Can you work these out from the model? Positions are in its coordinate system, mm. Face numbers are marked on the shaded views. A direction names the side the tool comes from. Round coordinates to 2 decimals unless told otherwise and drop trailing zeros. Loops run counter-clockwise (first coordinate to the right, second up) from the corner with the lowest first, then second, coordinate; pieces in that order, holes last. Notation, with made-up numbers: M -37,86 L 11,86 A26 cw 11,100 Z; hole C 24,72 d10. An arc over 180 degrees is marked long. Return JSON: item names as keys, results as strings.
Autodesk Inventor part; units mm, degrees
ref_plane "YZ Plane" through (0, 0, 0) normal (1, 0, 0) x (0, 1, 0)
ref_plane "XZ Plane" through (0, 0, 0) normal (0, 1, 0) x (-1, 0, 0)
ref_plane "XY Plane" through (0, 0, 0) normal (0, 0, 1) x (1, 0, 0)
sketch "Sketch1" plane through (0, 0, 0) normal (0, 1, 0) x (-1, 0, 0)
  line L0 (0, 0) -> (48.3, 0)
  line L1 (48.3, 0) -> (48.3, -15)
  line L2 (48.3, -15) -> (0, -15)
  line L3 (0, -15) -> (0, 0)
  circle A0 centre (48.3, 0) radius 1.5
  circle A1 centre (48.3, -15) radius 1.5
  line L4 (48.3, -15) -> (52.3, -15)
  line L5 (52.3, -15) -> (52.3, -17.5)
  line L6 (52.3, -17.5) -> (48.3, -17.5)
  line L7 (48.3, -17.5) -> (48.3, -15)
  line L8 (0, 0) -> (-4, 0)
  line L9 (-4, 0) -> (-4, 2.5)
  line L10 (-4, 2.5) -> (0, 2.5)
  line L11 (0, 2.5) -> (0, 0)
  line L12 (-4, 2.5) -> (52.3, 2.5)
  line L13 (52.3, 2.5) -> (52.3, -17.5)
  line L14 (52.3, -17.5) -> (-4, -17.5)
  line L15 (-4, -17.5) -> (-4, 2.5)
  line L16 (0, -2.5) -> (0, -12.5)
  circle A2 centre (0, -12.5) radius 2
  circle A3 centre (0, -2.5) radius 2
  point P0 (0, -7.5)
  dimension "d0" = 48.3
  dimension "d1" = 15
  dimension "d2" = 3
  dimension "d3" = 3
  dimension "d6" = 4
  dimension "d7" = 2.5
  dimension "d8" = 4
  dimension "d9" = 2.5
  dimension "d33" = 10
  dimension "d34" = 4
  dimension "d35" = 4
extrude "Extrusion1" add sketch "Sketch1" along normal blind 4 contours L11 L12 L13 L4 A1 L1 A0 L0 | L0 A0 L1 A1 L2 L3 A2 A3 | L3 A3 A2 L2 A1 L7 L14 L15 L8 | L8 L9 L10 L11 | L7 A1 L4 L5 L6
sketch "Sketch2" plane through (0, 4, 0) normal (0, 1, 0) x (1, 0, 0)
  line L0 (4, -2.5) -> (4, 17.5)
  line L1 (4, -2.5) -> (-14.15, -2.5)
  line L2 (-14.15, -2.5) -> (-14.15, 7.5)
  line L3 (-14.15, 7.5) -> (4, 7.5)
  line L4 (4, 7.5) -> (4, -2.5)
  circle A0 centre (-14.15, 7.5) radius 5
  circle A1 centre (-14.15, 7.5) radius 3.15
  point P0 (0, 0)
  dimension "d12" = 18.15
  dimension "d13" = 10
  dimension "d14" = 10
  dimension "d19" = 6.3
extrude "Extrusion2" add sketch "Sketch2" along normal blind 4 and the other way blind 2.5 contours A0 L2 A1 L3 | L3 A1 L2 A0
extrude "Extrusion3" cut sketch "Sketch2" against normal blind 4 contours A1 L2 L3 | L3 L2 A1
fillet "Fillet2" radius 4 1 edges at (-19.15, 4, -7.5)
sketch "Sketch3" plane through (0, 4, 0) normal (0, 1, 0) x (1, 0, 0)
  line L0 (4, 17.5) -> (-52.3, 17.5)
  line L1 (-52.3, 17.5) -> (-40.3, 17.5)
  line L2 (-40.3, 17.5) -> (-40.3, 12.5)
  line L3 (-40.3, 12.5) -> (-52.3, 12.5)
  line L4 (-52.3, 12.5) -> (-52.3, 17.5)
  line L5 (-52.3, -2.5) -> (4, -2.5)
  line L6 (-52.3, -2.5) -> (-40.3, -2.5)
  line L7 (-40.3, -2.5) -> (-40.3, 2.5)
  line L8 (-40.3, 2.5) -> (-52.3, 2.5)
  line L9 (-52.3, 2.5) -> (-52.3, -2.5)
  line L10 (-40.3, 2.5) -> (-25.3, 2.5)
  line L11 (-25.3, 2.5) -> (-25.3, 12.5)
  line L12 (-25.3, 12.5) -> (-40.3, 12.5)
  line L13 (-40.3, 12.5) -> (-40.3, 2.5)
  point P0 (0, 0)
  dimension "d25" = 12
  dimension "d26" = 5
  dimension "d27" = 12
  dimension "d28" = 5
  dimension "d29" = 15
extrude "Extrusion4" cut sketch "Sketch3" against normal blind 4 contours L12 L11 L10 L13
fillet "Fillet3" radius 2 4 edges at (-52.3, 2, 2.5) (4, 2, 2.5) (4, 2, -17.5) (-52.3, 2, -17.5)
sketch "Sketch4" plane through (0, 4, 0) normal (0, 1, 0) x (1, 0, 0)
  circle A0 centre (-48.3, 0) radius 1.5
  circle A1 centre (-48.3, 0) radius 1.5
  circle A2 centre (-48.3, 0) radius 2.5
  line L0 (-50.3, -2.5) -> (2, -2.5)
  circle A3 centre (-48.3, 15) radius 1.5
  circle A4 centre (-48.3, 15) radius 1.5
  circle A5 centre (-48.3, 15) radius 2.5
  line L1 (2, 17.5) -> (-50.3, 17.5)
  line L2 (-45.8, 12.5) -> (-52.3, 12.5)
  line L3 (-52.3, 12.5) -> (-52.3, 17.5)
  line L4 (-52.3, 17.5) -> (-45.8, 17.5)
  line L5 (-45.8, 17.5) -> (-45.8, 12.5)
  line L6 (-52.3, -2.5) -> (-45.8, -2.5)
  line L7 (-45.8, -2.5) -> (-45.8, 2.5)
  line L8 (-45.8, 2.5) -> (-52.3, 2.5)
  line L9 (-52.3, 2.5) -> (-52.3, -2.5)
  arc A6 (-52.3, -0.5) -> (-50.3, -2.5) centre (-50.3, -0.5) ccw
  circle A7 centre (-50.3, -0.5) radius 2
  arc A8 (-50.3, 17.5) -> (-52.3, 15.5) centre (-50.3, 15.5) ccw
  circle A9 centre (-50.3, 15.5) radius 2
  point P0 (0, 0)
  point P1 (-48.3, 12.5)
  point P2 (-45.8, 15)
  point P3 (-45.8, 0)
  point P4 (-48.3, 2.5)
extrude "Extrusion5" add sketch "Sketch4" along normal blind 3.5 contours A0 A7 A2 | A0 A7 A2 | A7 L9 L8 A2 | A2 A7 A6 | A2 L0 A7 | A2 L7 L0 | A3 A9 A5 | A3 A9 A5 | A9 L1 A5 | A5 A9 A8 | A5 L2 L3 A9 | L1 L5 A5
fillet "Fillet4" radius 2 6 edges at (-46.5322, 4, -13.2322) (-45.8, 4, -16.25) (-50.3, 4, -12.5) (-45.8, 4, 1.25) (-50.3, 4, -2.5) (-46.5322, 4, -1.7678)
properties part number "back_servo_support"
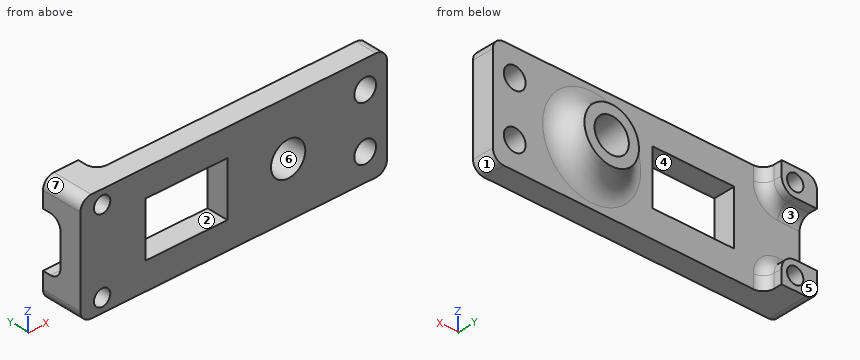
Q1. Suppose I cut it at C-C, the plane y = 1.75. Please give me the cut outline in (x, z), plus the area to 3 significant figures.
Results:
{"outline": "M -52.3,-15.5 A2 ccw -50.3,-17.5 L 2,-17.5 A2 ccw 4,-15.5 L 4,0.5 A2 ccw 2,2.5 L -50.3,2.5 A2 ccw -52.3,0.5 Z; hole C -48.3,-15 d3; hole C -48.3,0 d3; hole M -40.3,-12.5 L -25.3,-12.5 L -25.3,-2.5 L -40.3,-2.5 Z; hole C -14.15,-7.5 d6.3; hole C 0,-12.5 d4; hole C 0,-2.5 d4", "area": "902 mm2"}
Q2. On a 3-axis mill with a long thin cutter (end or side, diameter ignored), from which of +Z, -Z, +X, -X, +Y, -Y can I reach the whole of each face in a straight line? I mean the marked faces 1, 2 and 3. Say none if no direction works.
Results:
{"face 1": "-Z, +X, +Y, -Y", "face 2": "+Y, -Y", "face 3": "-X, +Y"}
Q3. If I drill on line 1 along Z through (x, y) = (-48.3, 6.35); line 2 along Z through (x, y) = (0, 1.4); line 3 along X through (y, z) = (1.75, -5.25), over which ranges is the centre line in solid material (lowest first)?
Results:
{"line 1": "z = -17.5 to -16.5, -13.5 to -12.5, -2.5 to -1.5, 1.5 to 2.5", "line 2": "z = -17.5 to -14.5, -10.5 to -4.5, -0.5 to 2.5", "line 3": "x = -52.3 to -40.3, -25.3 to -16.35, -11.95 to 4"}
Q4. Suppose I cut it at D-D, the plane y = 6.75. Please give me the cut outline in (x, z).
Results:
{"outline": "M -52.3,-15.5 A2 ccw -50.3,-17.5 L -45.8,-17.5 L -45.8,-15 A2.5 ccw -48.3,-12.5 L -52.3,-12.5 Z; M -52.3,-2.5 L -48.3,-2.5 A2.5 ccw -45.8,0 L -45.8,2.5 L -50.3,2.5 A2 ccw -52.3,0.5 Z; C -14.15,-7.5 d10.4; hole C -48.3,-15 d3; hole C -48.3,0 d3; hole C -14.15,-7.5 d6.3"}
Q5. Thinking about a two-plate mould opening in X: for the marked faces 4, 5, 6 and 7, which applies, pulls with the +X half, pulls with the -X half, needs draft (parallel to the pull), parting line crosses it, or undercut?
Results:
{"face 4": "undercut", "face 5": "needs draft", "face 6": "undercut", "face 7": "pulls with the -X half"}
Q6. I'm going to push flat-ended pins straight in: pin 1 Ø4 at (x, z) = (-14.15, -7.5) entering from +Y; pin 2 Ø0.8 at (y, z) = (6.5, 2) entering from +X; pin 3 Ø5.5 at (x, z) = (-49.5, 0) entering from +Y; pin 4 Ø0.8 at (x, y) = (-51.5, 6.5) entering from -Z. Where does each tip first touch, or does it pass through?
Results:
{"pin 1": "passes through", "pin 2": "stops at x = -45.8", "pin 3": "stops at y = 7.5", "pin 4": "stops at z = -17.33"}
Q7. Suppose I cut it at A-A, the plane z = -7.5. State how many separate pieces and enclosed holes the cut face has, plus the area to 3 significant figures.
Results:
{"separate pieces": "3", "enclosed holes": "0", "area": "162 mm2"}
